from build123d import *

# Parameters (mm, degrees)
SKETCH_R        = 4.5
PAD_DEPTH       = 7
SKETCH001_R     = 6
PAD001_DEPTH    = 5.8
SKETCH002_W     = 2
SKETCH002_H     = 10
POCKET_DEPTH    = 7
CHAMFER_SIZE    = 0.1
SKETCH003_W     = 2
SKETCH003_H     = 2
POCKET001_DEPTH = 5
POCKET002_DEPTH = 4


with BuildPart() as part:
    # Sketch → Pad (new body)
    with BuildSketch(Plane.XY):
        Circle(SKETCH_R)
    extrude(amount=PAD_DEPTH)

    # Sketch001 (on Face2 of Pad) → Pad001 (join)
    with BuildSketch(Plane(origin=(0, 0, 0), x_dir=(1, 0, 0), z_dir=(0, 0, -1))):
        Circle(SKETCH001_R)
    extrude(amount=PAD001_DEPTH)

    # Sketch002 (on Face2 of Pad001) → Pocket (cut)
    with BuildSketch(Plane.XY):
        with Locations((-6.4, 0)):
            Rectangle(SKETCH002_W, SKETCH002_H)
    extrude(amount=-POCKET_DEPTH, mode=Mode.SUBTRACT)

    # Chamfer
    chamfer_edges = [part.edges().sort_by_distance(p)[0] for p in [
        (-4.5, 0, 7),
    ]]
    chamfer(chamfer_edges, length=CHAMFER_SIZE)

    # Sketch003 (on Face3 of Chamfer) → Pocket001 (cut)
    with BuildSketch(Plane.XY):
        with Locations((0, 6)):
            Rectangle(SKETCH003_W, SKETCH003_H)
        with Locations((0, -6)):
            Rectangle(SKETCH003_W, SKETCH003_H)
    extrude(amount=-POCKET001_DEPTH, mode=Mode.SUBTRACT)

    # Sketch004 (on Face14 of Pocket001) → Pocket002 (cut)
    with BuildSketch(Plane(origin=(0, 0, -5.8), x_dir=(1, 0, 0), z_dir=(0, 0, -1))):
        with BuildLine():
            ThreePointArc((-4.559605, -2.5), (5.2, 0), (-4.559605, 2.5))
            Line((-4.559605, 2.5), (-4.559605, -2.5))
        make_face()
    extrude(amount=-POCKET002_DEPTH, mode=Mode.SUBTRACT)


solid = part.part
Here's how the part is built. I have some questions about the finished solid (model axes, mm). A direction names the side the tool comes from. Round coordinates to 2 decimals unless told otherwise and drop trailing zeros. Order: outer loops, then holes, each group sorted by start corner. A loop starts at its lowest first (then second) coordinate and runs counter-clockwise, first axis right, second up. Notation, with made-up numbers: (10, -38) -> (18, -38) arc R35 cw to (18, 1) -> close; hole circle Ø3 at (43.25, 33.5). An arc over 180 degrees is marked (long way). Return JSON: item names as keys, results as strings.
Q1. If we section it at C-C on y = 0: List the corners of the cut face in (x, z) for me.
Filled sheet:
{"outline": "(-5.4, -5.8) -> (-4.56, -5.8) -> (-4.56, -1.8) -> (5.2, -1.8) -> (5.2, -5.8) -> (6, -5.8) -> (6, 0) -> (4.5, 0) -> (4.5, 6.9) -> (4.4, 7) -> (-4.4, 7) -> (-4.5, 6.9) -> (-4.5, 0) -> (-5.4, 0) -> close"}
Q2. If we section it at A-A on x = 0: List the corners of the cut face in (y, z) for me, plus the area to 3 significant figures.
Filled sheet:
{"outline": "(-6, -5.8) -> (-5.2, -5.8) -> (-5.2, -5) -> (-6, -5) -> close; (-5, -1.8) -> (5, -1.8) -> (5, 0) -> (4.5, 0) -> (4.5, 6.9) -> (4.4, 7) -> (-4.4, 7) -> (-4.5, 6.9) -> (-4.5, 0) -> (-5, 0) -> close; (5.2, -5.8) -> (6, -5.8) -> (6, -5) -> (5.2, -5) -> close", "area": "82.3 mm^2"}
Q3. Which directions (+Z, -Z, +X, -X, +Y, -Y) give clear straight access to the entire face, cutting with the end or side of a thin tool? Please do faces 1 (the flat face through (0, -5, -1)), 2 (the flat face through (-1, -5.5, -2.5)), 3 (the flat face through (0, 0, -1.8)), 4 (the flat face through (1, 5.5, -2.5)), 5 (the flat face through (0, -5.5, -5)).
Filled sheet:
{"face 1": "+Z, -Z, -Y", "face 2": "+Z, -Y", "face 3": "-Z", "face 4": "+Z, +Y", "face 5": "+Z, +Y, -Y"}
Q4. If we mould it in two halves opening along Y, with no side actions, what happens to faces 6 (the cylindrical face through (4.22, 3.04, -3.83)), 7 (the cylindrical face through (-0.59, 4.46, 3.4)), 8 (the flat face through (-4.56, 0, -4)), 9 (the flat face through (3.2, 3.5, 0))? For each: released by +Y, released by -Y, zero draft, split by the parting line, or undercut.
Filled sheet:
{"face 6": "undercut", "face 7": "split by the parting line", "face 8": "undercut", "face 9": "zero draft"}
Q5. If we section it at B-B on z = -2: List the corners of the cut face in (x, y) for me.
Filled sheet:
{"outline": "(-5.4, -2.62) arc R6 ccw to (-1, -5.92) -> (-1, -5.1) arc R5.2 cw to (-4.56, -2.5) -> (-4.56, 2.5) arc R5.2 cw to (-1, 5.1) -> (-1, 5.92) arc R6 ccw to (-5.4, 2.62) -> close; (1, -5.92) arc R6 ccw to (1, 5.92) -> (1, 5.1) arc R5.2 cw to (1, -5.1) -> close"}
Q6. If we section it at D-D on z = 0.75: List the corners of the cut face in (x, y) for me.
Filled sheet:
{"outline": "circle Ø9 at (0, 0)"}
Q7. I need wall thicknesses on line 1 along X through (y, z) = (0, -4.45); line 2 along X through (y, z) = (1, -5); line 3 along Z through (x, y) = (0, 2.75). Which ranges of each line are inside material? Lowest first, please. Write a range as from..to.
Filled sheet:
{"line 1": "x = -5.4..-4.56, 5.2..6", "line 2": "x = -5.4..-4.56, 5.1..5.92", "line 3": "z = -1.8..7"}
Q8. For pin 1 Ø1.5 at (x, z) = (-1, -2.5) entering from +Y; pin 2 Ø4 at (x, z) = (1.5, -2) entering from -Y; pin 3 Ø1.2 at (y, z) = (1, -4) entering from +X, each with a flat end and sliding along its axis, tell me the tip position at first contact or that it passes through.
Filled sheet:
{"pin 1": "stops at y = 5.92", "pin 2": "stops at y = -5.92", "pin 3": "stops at x = 5.99"}
